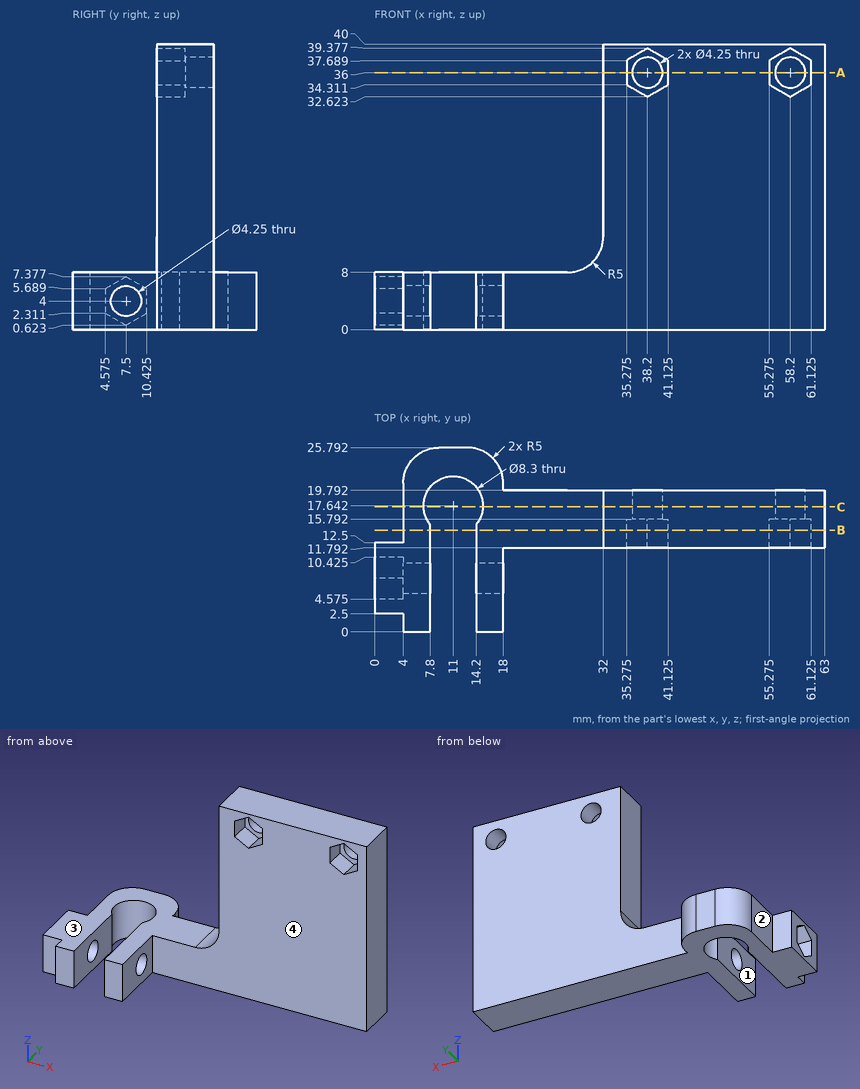
Input: dimensioned drawing with shaded views. Units: mm. Origin: part minimum x, y, z. A direction names the side the tool comes from. Coordinates: 2 decimals unless noted, no trailing zeros. Loops run counter-clockwise (first coordinate to the right, second up) from the corner with the lowest first, then second, coordinate; pieces in that order, holes last. Notation, with made-up numbers: M 20.25,49 L 52.25,49 A28 ccw 52.25,85 Z; hole C 7,40 d10. An arc over 180 degrees is marked long. One line per item, written item: value. Start each with the question number.
1) Reachability of the marked faces 1, 2, 3 and 4 from +Z, -Z, +X, -X, +Y, -Y: full face, straight path, thin tool, end or side. Return the list, or none.
2) Material intervals for L1, parallel to Z at x = 58.2, y = 19.05 (1 decimal); L2, parallel to X at y = 11.5, z = 2.5; L3, parallel to X at y = 17, z = 34.5 (1 decimal), sorted ascending. Write a range as from..to.
3) Cut plane C-C (y = 17.5). Count the separate pieces of the cut face and the enclosed holes in it, then the cut area to 3 significant figures.
4) Cut plane B-B (y = 14.25). Return loops of the section in (x, z) (1 decimal).
5) Pin query (flat end, axial travel): P1, Ø2.5, axis at y = 14, z = 36.5, coming from the -X side; P2, Ø4, axis at y = 5, z = 2.5, coming from the +X side; P3, Ø1, axis at x = 2.5, z = 4, coming from the +Y side. Return the tip coordinate at first contact, or that it passes through.
6) Cut plane A-A (z = 36). Return loops of the section in (x, y) (1 decimal), then the cut area to 3 significant figures.
Evaluation:
1. face 1: +Z, -Z, -Y
1. face 2: +Z, -Z, -X, +Y
1. face 3: +Z, -X, +Y, -Y
1. face 4: +Z, -Z, +X, -Y
2. L1: 0..33.9, 38.1..40
2. L2: 0..7.8, 14.2..18
2. L3: 32..36.7, 39.7..56.7, 59.7..63
3. separate pieces: 2
3. enclosed holes: 2
3. area: 1,370 mm^2
4. outline: M 4,0 L 7.8,0 L 7.8,8 L 4,8 Z; M 14.2,0 L 63,0 L 63,40 L 32,40 L 32,13 A5 cw 27,8 L 14.2,8 Z; hole M 35.3,34.3 L 38.2,32.6 L 41.1,34.3 L 41.1,37.7 L 38.2,39.4 L 35.3,37.7 Z; hole M 55.3,34.3 L 58.2,32.6 L 61.1,34.3 L 61.1,37.7 L 58.2,39.4 L 55.3,37.7 Z
5. P1: x = 32
5. P2: x = 18
5. P3: y = 12.5
6. outline: M 32,11.8 L 35.3,11.8 L 35.3,15.8 L 36.1,15.8 L 36.1,19.8 L 32,19.8 Z; M 40.3,15.8 L 41.1,15.8 L 41.1,11.8 L 55.3,11.8 L 55.3,15.8 L 56.1,15.8 L 56.1,19.8 L 40.3,19.8 Z; M 60.3,15.8 L 61.1,15.8 L 61.1,11.8 L 63,11.8 L 63,19.8 L 60.3,19.8 Z
6. area: 167 mm^2
